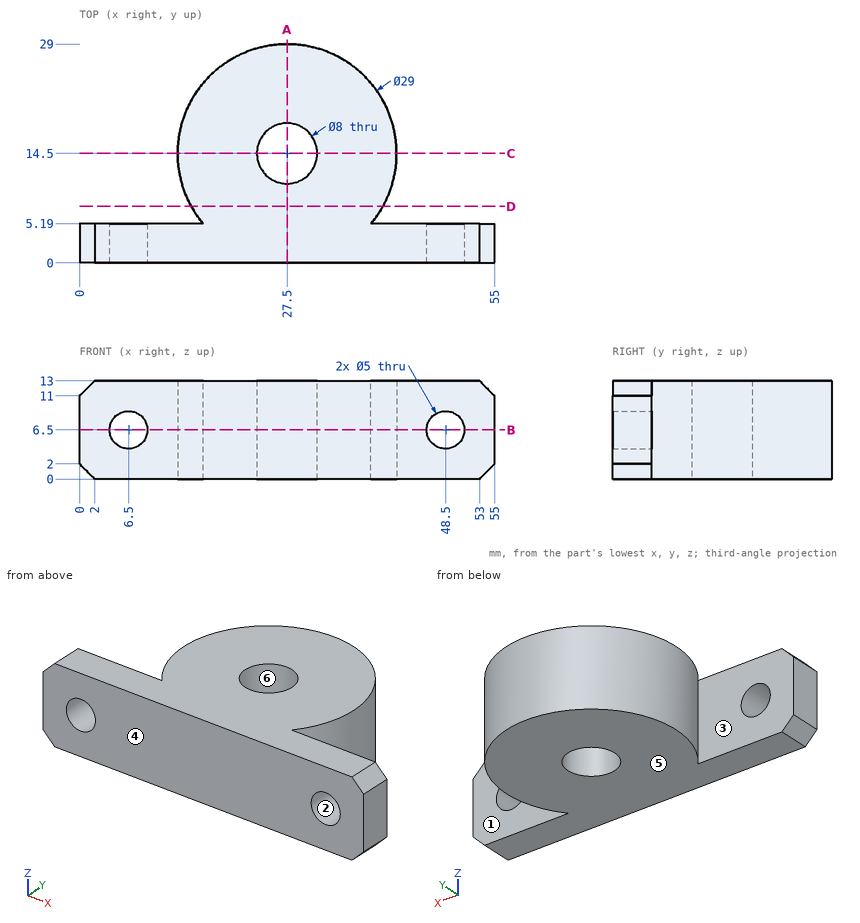
Could you check a few things on this drawing? It's one solid part, dimensions in mm from its lowest x, y, z. A direction names the side the tool comes from. Give positions to 0.01 mm unless a question says otherwise; leave off trailing zeros. Order: outer loops, then holes, each group sorted by start corner. A loop starts at its lowest first (then second) coordinate and runs counter-clockwise, first axis right, second up. Notation, with made-up numbers: (47.5, -22.75) -> (88.5, -22.75) arc R29 ccw to (88.5, 1.25) -> close; hole circle Ø10 at (74, -25). An arc over 180 degrees is marked (long way). Answer in a Markdown table with one row per item. Add a question column.
Item 1: For the marked faces 1, 2 and 3, which set-ups out of +Z, -Z, +X, -X, +Y, -Y let a thin tool reach every point of the face, with its end or its side?
Item 2: Imagine slicing it at D-D (y = 7.5). List the corners of the cut face in (x, z) for me, and give its area (3 significant figures).
Item 3: Please list where these lines run through material, in increasing order: probe 1 along Z at (x, y) = (6.5, 1.6); probe 2 along X at (y, z) = (3.25, 7); probe 3 along Y at (x, z) = (25.5, 3.5).
Item 4: I'm going to push flat-ended pins straight in: P1, Ø4, axis at y = 14, z = 10, coming from the +X side; P2, Ø10, axis at x = 46.5, y = 23, coming from the +Z side; P3, Ø4, axis at x = 46, z = 7.5, coming from the +Y side; P4, Ø4, axis at x = 22.5, z = 9, coming from the +Y side. Where does each tip first touch, or does it pass through?
Item 5: We'd pull the mould along Y, two halves only. Please class the marked faces 4, 5 and 6: pulls with the +Y half, pulls with the -Y half, needs draft (parallel to the pull), parting line crosses it, or undercut.
Item 6: Imagine slicing it at B-B (z = 6.5). List the corners of the cut face in (x, y) for me.
Item 7: Imagine slicing it at C-C (y = 14.5). List the corners of the cut face in (x, z) for me.
Item 8: Imagine slicing it at A-A (x = 27.5). List the corners of the cut face in (y, z) for me.
Result:
| question | item | result |
|---|---|---|
| 1 | face 1 | +Z, -Z, +X |
| 1 | face 2 | +Y, -Y |
| 1 | face 3 | +Z, -Z, -X |
| 2 | outline | (14.8, 0) -> (40.2, 0) -> (40.2, 13) -> (14.8, 13) -> close |
| 2 | area | 330 mm2 |
| 3 | probe 1 | 0 to 4, 9 to 13 |
| 3 | probe 2 | 0 to 4.05, 8.95 to 46.05, 50.95 to 55 |
| 3 | probe 3 | 0 to 11.04, 17.96 to 28.86 |
| 4 | P1 | x = 42 |
| 4 | P2 | through |
| 4 | P3 | y = 5.19 |
| 4 | P4 | y = 28.69 |
| 5 | face 4 | pulls with the -Y half |
| 5 | face 5 | needs draft |
| 5 | face 6 | undercut |
| 6 | outline | (0, 0) -> (4, 0) -> (4, 5.19) -> (0, 5.19) -> close; (9, 0) -> (46, 0) -> (46, 5.19) -> (38.62, 5.19) arc R14.5 ccw (long way) to (16.38, 5.19) -> (9, 5.19) -> close; (51, 0) -> (55, 0) -> (55, 5.19) -> (51, 5.19) -> close; hole circle Ø8 at (27.5, 14.5) |
| 7 | outline | (13, 0) -> (23.5, 0) -> (23.5, 13) -> (13, 13) -> close; (31.5, 0) -> (42, 0) -> (42, 13) -> (31.5, 13) -> close |
| 8 | outline | (0, 0) -> (10.5, 0) -> (10.5, 13) -> (0, 13) -> close; (18.5, 0) -> (29, 0) -> (29, 13) -> (18.5, 13) -> close |
